CAD build for the part. Positions are in the model's coordinates, mm. Round coordinates to 2 decimals unless told otherwise and drop trailing zeros. Order: outer loops, then holes, each group sorted by start corner. A loop starts at its lowest first (then second) coordinate and runs counter-clockwise, first axis right, second up. Notation, with made-up numbers: M -31.75,40 L -2.75,40 A36 ccw -2.75,74 Z; hole C 24,31.25 d9. An arc over 180 degrees is marked long. Answer as a JSON object with one key per item and string values.
```python
from build123d import *

# Parameters (mm, degrees)
PAD011_DEPTH           = 32
SKETCH048_R            = 6
POCKET006_DEPTH        = 331.323772
LINEARPATTERN004_COUNT = 4
LINEARPATTERN004_PITCH = 200


with BuildPart() as part:
    # Sketch047 → Pad011 (new body)
    with BuildSketch(Plane.XY):
        Polygon((-556.862366, 411.885088), (10.320579, 14.739314), (13.762038, 19.654226), (-553.420907, 416.8), align=None)
    extrude(amount=PAD011_DEPTH)

    # Sketch048 (on Face1 of Pad011) → Pocket006 (cut, through all)
    with BuildSketch(Plane(origin=(10.320579, 14.739314, 0), x_dir=(0.819152, -0.573576, 0), z_dir=(-0.573576, -0.819152, 0))):
        with Locations((-672.402526, 16)):
            Circle(SKETCH048_R)
    pocket006 = extrude(amount=-POCKET006_DEPTH, mode=Mode.SUBTRACT)

    # LinearPattern004: Pocket006 ×4
    with Locations(*[Vector(0.819152, -0.573576, 0) * (i * LINEARPATTERN004_PITCH) for i in range(1, LINEARPATTERN004_COUNT)]):
        add(pocket006, mode=Mode.SUBTRACT)


with BuildPart() as part_1:
    # Body008 placement: moved
    add(part.part.moved(Location((0, 0, 9))))


solid = part_1.part
```
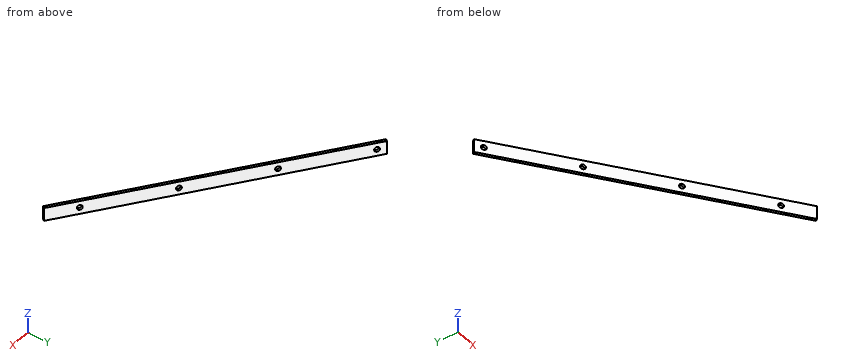
Item 1: Saw through at B-B on y = 41. List the corners of the cut face in (x, z), and give its area (3 significant figures).
Worked answers:
{"outline": "M -27.18,9 L -16.72,9 L -16.72,41 L -27.18,41 Z", "area": "335 mm2"}
Item 2: Drop flat-ended pins along their axis: pin 1 Ø1 at (y, z) = (97.5, 12.5) entering from +X; pin 2 Ø12 at (x, z) = (-413.5, 14) entering from +Y; pin 3 Ø1 at (y, z) = (141.5, 36.5) entering from -X. Give the stop position or say it passes through.
Worked answers:
{"pin 1": "stops at x = -96.7", "pin 2": "stops at y = 323.03", "pin 3": "stops at x = -171.43"}
Item 3: Saw through at A-A on x = -83.5. List the corners of the cut face in (y, z).
Worked answers:
{"outline": "M 80.43,9 L 87.76,9 L 87.76,41 L 80.43,41 Z"}
Item 4: Wall check: line 1 along Z through (x, y) = (-379.5, 288); line 2 along X through (y, z) = (243, 16.5); line 3 along Y through (x, z) = (-490, 37). Give the ranges that are in metal, low to high. Write a range as [from, to].
Worked answers:
{"line 1": "z = [9, 20.24], [29.76, 41]", "line 2": "x = [-315.67, -305.21]", "line 3": "y = [365.07, 372.39]"}
